```python
from build123d import *

# Parameters (mm, degrees)
ESBO_O1_W                = 103
ESBO_O1_H                = 153
RESSALTO_EXTRUS_O1_DEPTH = 3
ESBO_O2_W                = 32
ESBO_O2_H                = 12
CORTE_EXTRUS_O1_DEPTH    = 93.268629555
FILETE1_R                = 3
ESBO_O3_W                = 33
ESBO_O3_H                = 3
CORTE_EXTRUS_O2_DEPTH    = 93.268629555
ESBO_O4_W                = 3
ESBO_O4_H                = 27
ESBO_O4_R                = 1.5
CORTE_EXTRUS_O3_DEPTH    = 93.268629555


with BuildPart() as part:
    # Esboço1 → Ressalto-extrusão1 (new body)
    with BuildSketch(Plane.XY):
        Rectangle(ESBO_O1_W, ESBO_O1_H)
    extrude(amount=RESSALTO_EXTRUS_O1_DEPTH)

    # Esboço2 → Corte-extrusão1 (cut, through all)
    with BuildSketch(Plane.XY.offset(3)):
        with Locations((0, -32)):
            Rectangle(ESBO_O2_W, ESBO_O2_H)
    extrude(amount=-CORTE_EXTRUS_O1_DEPTH, mode=Mode.SUBTRACT)

    # Filete1
    filete1_edges = [part.edges().sort_by_distance(p)[0] for p in [
        (16, -26, 1.5),
        (16, -38, 1.5),
        (-16, -38, 1.5),
        (-16, -26, 1.5),
    ]]
    fillet(filete1_edges, radius=FILETE1_R)

    # Esboço3 → Corte-extrusão2 (cut, through all)
    with BuildSketch(Plane(origin=(0, 0, 0), x_dir=(-1, 0, 0), z_dir=(0, 0, -1))):
        with Locations((35, -75)):
            Rectangle(ESBO_O3_W, ESBO_O3_H)
        with Locations((-35, -75)):
            Rectangle(ESBO_O3_W, ESBO_O3_H)
        with Locations((35, 75)):
            Rectangle(ESBO_O3_W, ESBO_O3_H)
        with Locations((-35, 75)):
            Rectangle(ESBO_O3_W, ESBO_O3_H)
    extrude(amount=-CORTE_EXTRUS_O2_DEPTH, mode=Mode.SUBTRACT)

    # Esboço4 → Corte-extrusão3 (cut, through all)
    with BuildSketch(Plane(origin=(0, 0, 0), x_dir=(-1, 0, 0), z_dir=(0, 0, -1))):
        with Locations((50, 60)):
            Rectangle(ESBO_O4_W, ESBO_O4_H)
        with Locations((50, -60)):
            Rectangle(ESBO_O4_W, ESBO_O4_H)
        with Locations((-50, -60)):
            Rectangle(ESBO_O4_W, ESBO_O4_H)
        with Locations((-50, 60)):
            Rectangle(ESBO_O4_W, ESBO_O4_H)
        with Locations((-6.5, -66.5)):
            Circle(ESBO_O4_R)
        with Locations((-6.5, -56.5)):
            Circle(ESBO_O4_R)
        with Locations((6.5, -66.5)):
            Circle(ESBO_O4_R)
        with Locations((6.5, -56.5)):
            Circle(ESBO_O4_R)
    extrude(amount=-CORTE_EXTRUS_O3_DEPTH, mode=Mode.SUBTRACT)


solid = part.part
```
Geometry: final body of the model. Coordinates: model frame, mm. A direction names the side the tool comes from. Coordinates: 2 decimals unless noted, no trailing zeros. Order: outer loops, then holes, each group sorted by start corner. A loop starts at its lowest first (then second) coordinate and runs counter-clockwise, first axis right, second up. Notation, with made-up numbers: (-23, 26.25) -> (33, 26.25) arc R13 ccw to (33, 40.25) -> close; hole circle Ø1 at (16, 43). An arc over 180 degrees is marked (long way). Answer in a Markdown table with one row per item.
Item 1: Section D-D on x = 38.5. Output: boundary loops of the cut face in (y, z).
Return value:
| item | result |
|---|---|
| outline | (-73.5, 0) -> (73.5, 0) -> (73.5, 3) -> (-73.5, 3) -> close |
Item 2: Access query for faces 1 (the flat face through (-33, -73.5, 1)), 2 (the flat face through (50, 46.5, 1)), 3 (the flat face through (-18.5, 75, 1)). Directions: +Z, -Z, +X, -X, +Y, -Y. A direction counts if a zero-diameter tool reaches every point of the face in a straight line with its end or side. Return the directions, or none.
Return value:
| item | result |
|---|---|
| face 1 | +Z, -Z, -X, -Y |
| face 2 | +Z, -Z, +X, +Y |
| face 3 | +Z, -Z, -X, +Y |
Item 3: Section B-B on x = -6.5. Output: boundary loops of the cut face in (y, z), plus the area to 3 significant figures.
Return value:
| item | result |
|---|---|
| outline | (-76.5, 0) -> (-68, 0) -> (-68, 3) -> (-76.5, 3) -> close; (-65, 0) -> (-58, 0) -> (-58, 3) -> (-65, 3) -> close; (-55, 0) -> (-38, 0) -> (-38, 3) -> (-55, 3) -> close; (-26, 0) -> (76.5, 0) -> (76.5, 3) -> (-26, 3) -> close |
| area | 405 mm² |
Item 4: Ray query, L1, parallel to Y at x = -6.5, z = 1.4; L2, parallel to X at y = -66.5, z = 1.6; L3, parallel to Y at x = 27, z = 2.3. Return the intervals inside material, ascending.
Return value:
| item | result |
|---|---|
| L1 | y = -76.5 to -68, -65 to -58, -55 to -38, -26 to 76.5 |
| L2 | x = -48.5 to -8, -5 to 5, 8 to 48.5 |
| L3 | y = -73.5 to 73.5 |
Item 5: Section C-C on y = -56.5. Output: boundary loops of the cut face in (x, z).
Return value:
| item | result |
|---|---|
| outline | (-48.5, 0) -> (-8, 0) -> (-8, 3) -> (-48.5, 3) -> close; (-5, 0) -> (5, 0) -> (5, 3) -> (-5, 3) -> close; (8, 0) -> (48.5, 0) -> (48.5, 3) -> (8, 3) -> close |
Item 6: Contact query for flat-ended pins moving along their axis: P1, Ø1.5, axis at x = 49.5, z = 1.5, coming from the +Y side; P2, Ø6, axis at x = -24.5, y = 32.5, coming from the -Z side; P3, Ø0.9, axis at y = -75, z = 1, coming from the +X side; P4, Ø1.5, axis at x = 32.5, z = 2, coming from the -Y side. Output: stop coordinate, or through.
Return value:
| item | result |
|---|---|
| P1 | stops at y = 46.5 |
| P2 | stops at z = 0 |
| P3 | stops at x = 18.5 |
| P4 | stops at y = -73.5 |
Item 7: Section A-A on z = 0.95. State how many separate pieces and enclosed holes the cut face has, plus the area to 3 significant figures.
Return value:
| item | result |
|---|---|
| separate pieces | 1 |
| enclosed holes | 5 |
| area | 14,600 mm² |
Item 8: Draft query along Y for faces 4 (the flat face through (0, -26, 2)), 5 (the flat face through (-1, 1, 3)), 6 (the flat face through (0, -76.5, 1)). Return one class per face: released by +Y, released by -Y, zero draft, split by the parting line, or undercut.
Return value:
| item | result |
|---|---|
| face 4 | undercut |
| face 5 | zero draft |
| face 6 | released by -Y |
